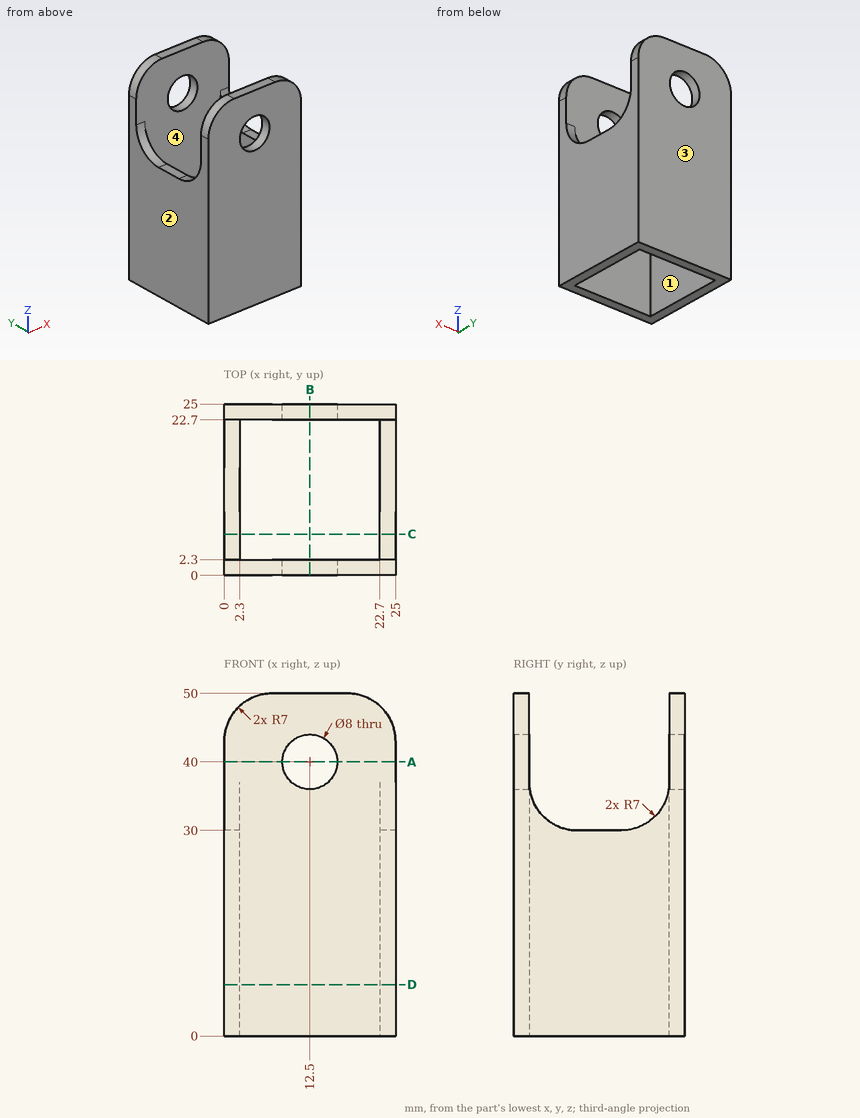
Geometry check sheet. Reference: drawing and pictorial views, mm from the part's lowest x, y, z. Coordinates: 2 decimals unless noted, no trailing zeros. Order: outer loops, then holes, each group sorted by start corner. A loop starts at its lowest first (then second) coordinate and runs counter-clockwise, first axis right, second up.
Item 1: Scan lines: line 1 along X through (y, z) = (16, 4.5); line 2 along X through (y, z) = (24.1, 40). Record each from-to range of solid material in increasing order.
Item 2: Section check D-D (z = 7.5). Enter the section's corners in (x, y).
Item 3: Section check A-A (z = 40). Enter the section's corners in (x, y).
Item 4: Section check B-B (x = 12.5). Enter the section's corners in (y, z).
Item 5: Mould release check, pull along X, two halves, no side actions. Record for the marked faces 1, 2, 3 and 4: released by +X, released by -X, zero draft, split by the parting line, or undercut.
Item 6: Depth check by flat-ended pin: pin 1 (2.5 mm diameter, centred on x = 23.5, y = 12.5, fed in from +Z). Enter the tip coordinate at first touch or a pass-through.
Item 7: Section check C-C (y = 6). Enter the section's corners in (x, z).
Check sheet entries:
1. line 1: x = 0 to 2.3, 22.7 to 25
1. line 2: x = 0 to 8.5, 16.5 to 25
2. outline: (0, 0) - (25, 0) - (25, 25) - (0, 25) - close; hole (2.3, 2.3) - (22.7, 2.3) - (22.7, 22.7) - (2.3, 22.7) - close
3. outline: (0, 0) - (8.5, 0) - (8.5, 2.3) - (0, 2.3) - close; (0, 22.7) - (8.5, 22.7) - (8.5, 25) - (0, 25) - close; (16.5, 0) - (25, 0) - (25, 2.3) - (16.5, 2.3) - close; (16.5, 22.7) - (25, 22.7) - (25, 25) - (16.5, 25) - close
4. outline: (0, 0) - (2.3, 0) - (2.3, 36) - (0, 36) - close; (0, 44) - (2.3, 44) - (2.3, 50) - (0, 50) - close; (22.7, 0) - (25, 0) - (25, 36) - (22.7, 36) - close; (22.7, 44) - (25, 44) - (25, 50) - (22.7, 50) - close
5. face 1: undercut
5. face 2: released by -X
5. face 3: zero draft
5. face 4: undercut
6. pin 1: stops at z = 30
7. outline: (0, 0) - (2.3, 0) - (2.3, 30.83) - (0, 30.83) - close; (22.7, 0) - (25, 0) - (25, 30.83) - (22.7, 30.83) - close
